Work out the finished part from the listing and answer in its coordinate system (mm). Face numbers are marked on the shaded views. Coordinates: 2 decimals unless noted, no trailing zeros. Loops run counter-clockwise (first coordinate to the right, second up) from the corner with the lowest first, then second, coordinate; pieces in that order, holes last. Notation, with made-up numbers: (-3, -31) -> (40, -31) arc R20 cw to (40, 6) -> close; hole circle Ø3 at (43.5, 3.25). An arc over 180 degrees is marked (long way). One line per question, with ' | ' between items.
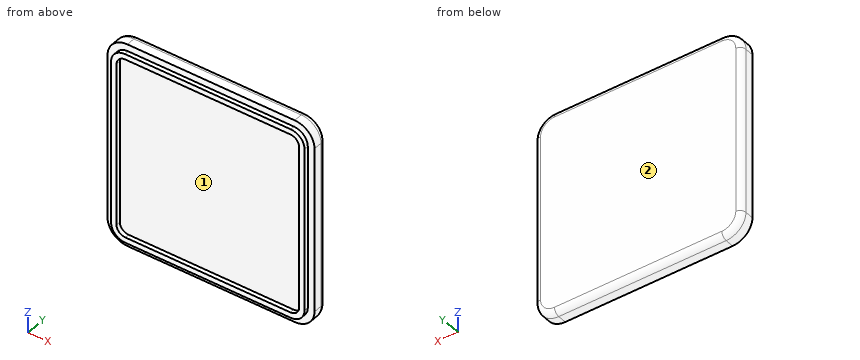
Autodesk Fusion 360 part; units mm, degrees
sketch "Sketch1" plane through (0, 0, 0) normal (0, 1, 0) x (1, 0, 0)
  line L0 (35.25, -35.25) -> (-35.25, -35.25)
  line L1 (-35.25, -35.25) -> (-35.25, 35.25)
  line L2 (-35.25, 35.25) -> (35.25, 35.25)
  line L3 (35.25, 35.25) -> (35.25, -35.25)
  line L4 (35.25, -35.25) -> (-35.25, 35.25) construction
  line L5 (-35.25, -35.25) -> (35.25, 35.25) construction
  dimension "d1" = 70.5
  dimension "d2" = 70.5
extrude "Extrude1" add sketch "Sketch1" along normal blind 5
sketch "Sketch2" plane through (0, 0, 0) normal (0, -1, 0) x (1, 0, 0)
  line L0 (-35.25, -35.25) -> (35.25, -35.25)
  line L1 (35.25, -35.25) -> (35.25, 35.25)
  line L2 (35.25, 35.25) -> (-35.25, 35.25)
  line L3 (-35.25, 35.25) -> (-35.25, -35.25)
  line L4 (32.95, -32.95) -> (32.95, 32.95)
  line L5 (32.95, 32.95) -> (-32.95, 32.95)
  line L6 (-32.95, 32.95) -> (-32.95, -32.95)
  line L7 (-32.95, -32.95) -> (32.95, -32.95)
  line L8 (32.95, 0) -> (30.95, 0)
  line L9 (0, -32.95) -> (0, -30.95)
  line L10 (-32.95, 0) -> (-30.95, 0)
  line L11 (0, 32.95) -> (0, 30.95)
  line L12 (-31.1, 31.1) -> (31.1, 31.1)
  line L13 (31.1, 31.1) -> (31.1, -31.1)
  line L14 (31.1, -31.1) -> (-31.1, -31.1)
  line L15 (-31.1, -31.1) -> (-31.1, 31.1)
  dimension "d5" = -2.3
  dimension "d6" = 2
  dimension "d7" = 2
  dimension "d8" = 2
  dimension "d9" = 2
extrude "Extrude2" add sketch "Sketch2" along normal blind 1.5 contours L4 L7 L8 L9 L13 L14 | L4 L5 L8 L11 L12 L13 | L6 L7 L9 L10 L14 L15 | L5 L6 L10 L11 L12 L15
fillet "Fillet1" radius 4.75 4 edges at (-32.95, -0.75, 32.95) (32.95, -0.75, 32.95) (32.95, -0.75, -32.95) (-32.95, -0.75, -32.95)
fillet "Fillet2" radius 3 4 edges at (31.1, -0.75, 31.1) (-31.1, -0.75, 31.1) (31.1, -0.75, -31.1) (-31.1, -0.75, -31.1)
fillet "Fillet3" radius 6.75 4 edges at (-35.25, 2.5, 35.25) (35.25, 2.5, 35.25) (35.25, 2.5, -35.25) (-35.25, 2.5, -35.25)
fillet "Fillet4" radius 2 8 edges at (-33.273, 5, -33.273) (-35.25, 5, 0) (-33.273, 5, 33.273) (0, 5, 35.25) (33.273, 5, 33.273) (35.25, 5, 0) (33.273, 5, -33.273) (0, 5, -35.25)
1) Find section A-A (z = 19). Write down the section's boundary in (x, y).
Check values:
outline: (-35.25, 0) -> (-32.95, 0) -> (-32.95, -1.5) -> (-31.1, -1.5) -> (-31.1, 0) -> (31.1, 0) -> (31.1, -1.5) -> (32.95, -1.5) -> (32.95, 0) -> (35.25, 0) -> (35.25, 3) arc R2 ccw to (33.25, 5) -> (-33.25, 5) arc R2 ccw to (-35.25, 3) -> close
2) Find section B-B (x = 21.5). Write down the section's boundary in (y, z).
Check values:
outline: (-1.5, -32.95) -> (0, -32.95) -> (0, -35.25) -> (3, -35.25) arc R2 ccw to (5, -33.25) -> (5, 33.25) arc R2 ccw to (3, 35.25) -> (0, 35.25) -> (0, 32.95) -> (-1.5, 32.95) -> (-1.5, 31.1) -> (0, 31.1) -> (0, -31.1) -> (-1.5, -31.1) -> close
3) Find the intervals of material crossed by line 1 along Z through (x, y) = (19, -0.5); line 2 along Z through (x, y) = (-3.5, 3.25), in increasing order.
Check values:
line 1: z = -32.95 to -31.1, 31.1 to 32.95 | line 2: z = -35.23 to 35.23
4) Flat-ended cylindrical pins translate along their axes: pin 1 (1.6 mm diameter, centred on x = 6, y = -1, fed in from +Z); pin 2 (10 mm diameter, centred on x = 2.5, z = -8.5, fed in from -Y); pin 3 (0.8 mm diameter, centred on y = -1, z = 4, fed in from +X). Find the tip coordinate at first contact, or state that the pin passes through.
Check values:
pin 1: stops at z = 32.95 | pin 2: stops at y = 0 | pin 3: stops at x = 32.95
5) The mould has two halves that part along X. Classify the marked faces 1 and 2: released by +X, released by -X, zero draft, split by the parting line, or undercut.
Check values:
face 1: undercut | face 2: zero draft
